Autodesk Fusion 360 part; units mm, degrees
sketch "Sketch1" plane through (0, 0, 0) normal (1, 0, 0) x (0, 1, 0)
  line L0 (90, -90) -> (90, 90)
  line L1 (-95, 95) -> (95, -95) construction
  line L2 (95, 95) -> (-95, 95)
  line L3 (85, 85) -> (-85, 85)
  line L4 (-85, -85) -> (85, -85)
  line L5 (85, -85) -> (85, 85)
  line L6 (-95, 95) -> (-95, -95)
  line L7 (0, 85) -> (0, -85) construction
  line L8 (-85, 85) -> (-85, -85)
  line L9 (95, 95) -> (-95, -95) construction
  line L10 (95, -95) -> (95, 95)
  line L11 (90, 90) -> (-90, 90)
  line L12 (-90, -90) -> (90, -90)
  line L13 (-85, 0) -> (85, 0) construction
  line L14 (-95, -95) -> (95, -95)
  line L15 (-90, 90) -> (-90, -90)
  dimension "d3" = -5
  dimension "d4" = -5
  dimension "d5" = 190
  dimension "d6" = 190
extrude "Extrude4" add sketch "Sketch1" along normal mid plane 50 contours L0 L11 L12 L15
extrude "Extrude5" add sketch "Sketch1" along normal mid plane 60 contours L2 L6 L10 L14
sketch "Sketch2" plane through (0, 0, -85) normal (0, 0, 1) x (-1, 0, 0)
  line L0 (25, 85) -> (-25, 85)
  line L1 (-25, 85) -> (-25, -85)
  line L2 (-25, -85) -> (25, -85)
  line L3 (25, -85) -> (25, 85)
  line L4 (-2.525, 85) -> (2.525, 85)
  line L5 (2.525, 85) -> (2.525, -85)
  line L6 (2.525, -85) -> (-2.525, -85)
  line L7 (-2.525, -85) -> (-2.525, 85)
  line L8 (-2.525, 85) -> (2.525, -85) construction
  line L9 (2.525, 85) -> (-2.525, -85) construction
  line L10 (5.025, 87.5) -> (5.025, -87.5)
  line L11 (5.025, -87.5) -> (-5.025, -87.5)
  line L12 (-5.025, -87.5) -> (-5.025, 87.5)
  line L13 (-5.025, 87.5) -> (5.025, 87.5)
  dimension "d39" = -2.5
  dimension "d40" = 5.05
extrude "Extrude6" add sketch "Sketch2" along normal blind 5 contours L0 L2 L5 L10 | L0 L2 L7 L12
sketch "Sketch3" plane through (0, 0, 85) normal (0, 0, -1) x (1, 0, 0)
  line L0 (-25, -85) -> (25, -85)
  line L1 (25, -85) -> (25, 85)
  line L2 (25, 85) -> (-25, 85)
  line L3 (-25, 85) -> (-25, -85)
  line L4 (-2.5, 85) -> (2.5, 85)
  line L5 (2.5, 85) -> (2.5, -85)
  line L6 (2.5, -85) -> (-2.5, -85)
  line L7 (-2.5, -85) -> (-2.5, 85)
  line L8 (-2.5, 85) -> (2.5, -85) construction
  line L9 (2.5, 85) -> (-2.5, -85) construction
  line L10 (5, 87.5) -> (5, -87.5)
  line L11 (5, -87.5) -> (-5, -87.5)
  line L12 (-5, -87.5) -> (-5, 87.5)
  line L13 (-5, 87.5) -> (5, 87.5)
  dimension "d43" = 5
  dimension "d44" = -2.5
extrude "Extrude7" add sketch "Sketch3" along normal blind 5 contours L0 L2 L7 L12 | L0 L2 L5 L10
equation "d6 = d5"
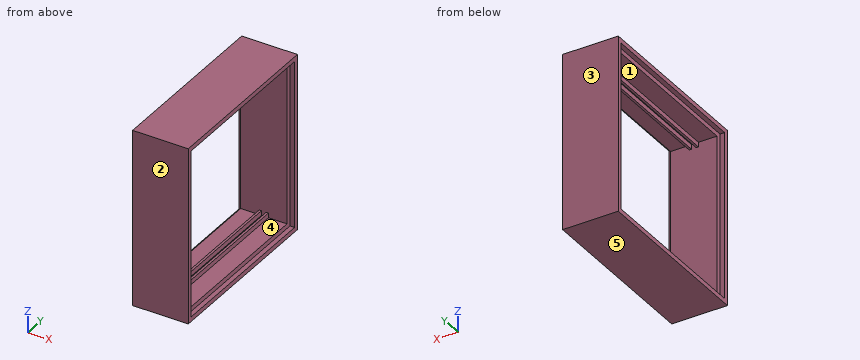
Input: part model. Units: mm. Frame: model coordinates. Face numbers are marked on the shaded views. A direction names the side the tool comes from. Coordinates: 2 decimals unless noted, no trailing zeros. Write each loop counter-clockwise with the first axis right and the second up, starting at its lowest first coordinate (ties: lowest second). Pieces come first, ordered by that corner, then holes.
1) Material intervals for line 1 along Z through (x, y) = (26, 26.5); line 2 along X through (y, z) = (40, 83.5); line 3 along Y through (x, z) = (10.5, 68), sorted ascending.
2) Section A-A on z = 75.5. Output: boundary loops of the cut face in (x, y), and give its area (3 significant figures).
3) Set-up query: the marked faces 1 and 2. Return all of +Z, -Z, +X, -X, +Y, -Y with unobstructed straight access to the full face (end or side cutting, diameter ignored); none if empty.
4) Pin query (flat end, axial travel): pin 1 Ø1.5 at (y, z) = (-18.5, -82.5) entering from -X (3 decimals); pin 2 Ø5.5 at (y, z) = (9.5, 82.5) entering from -X; pin 3 Ø5.5 at (y, z) = (-3.5, 81.5) entering from +X. Return the tip coordinate at first contact, or that it passes through.
5) Section C-C on x = -20. Output: boundary loops of the cut face in (y, z), and give its area (3 significant figures).
6) Mould query, pull axis Y, two halves, no side actions, for the marked faces 3, 4 and 5. Classes: pulls with the +Y half, pulls with the -Y half, needs draft (parallel to the pull), parting line crosses it, or undercut.
Check result:
1. line 1: z = -95 to -90, 90 to 95
1. line 2: x = -5 to -2.5, 2.5 to 5
1. line 3: y = -95 to -85, 85 to 95
2. outline: (-30, -95) - (30, -95) - (30, -90) - (25, -90) - (25, -85) - (-25, -85) - (-25, -90) - (-30, -90) - close; (-30, 90) - (-25, 90) - (-25, 85) - (25, 85) - (25, 90) - (30, 90) - (30, 95) - (-30, 95) - close
2. area: 1,100 mm2
3. face 1: -X
3. face 2: +Z, -Z, +X, -X, -Y
4. pin 1: stops at x = -5.025
4. pin 2: stops at x = -25
4. pin 3: stops at x = 5
5. outline: (-95, -95) - (95, -95) - (95, 95) - (-95, 95) - close; hole (-85, -85) - (85, -85) - (85, 85) - (-85, 85) - close
5. area: 7,200 mm2
6. face 3: pulls with the +Y half
6. face 4: undercut
6. face 5: needs draft
